from build123d import *

# Parameters (mm, degrees)
CUT_EXTRUDE1_DEPTH      = 64.162373268
CUT_EXTRUDE1_DEPTH_BACK = 64.162373268
SKETCH2_R               = 5
CUT_EXTRUDE2_DEPTH      = 63.964159794
CUT_EXTRUDE2_DEPTH_BACK = 63.964159794
SKETCH3_R               = 5


with BuildPart() as part:
    # Sketch1 → Revolve1 (revolve)
    with BuildSketch(Plane.XY, mode=Mode.PRIVATE) as revolve1_sk:
        Polygon((11.25, 0), (11.25, 12), (18, 12), (27.357798165, 42), (33.357798165, 42), (22.5, 0), align=None)
    revolve(revolve1_sk.sketch.rotate(Axis((0, 40.458715596, 0), (0, -1, 0)), 90), axis=Axis((0, 40.458715596, 0), (0, -1, 0)))

    # Sketch2 → Cut-Extrude1 (cut, two sides: drawn at the far end of the back side and taken through both)
    with BuildSketch(Plane.XY.offset(-CUT_EXTRUDE1_DEPTH_BACK)):
        with Locations((0, 42)):
            Circle(SKETCH2_R)
    extrude(amount=CUT_EXTRUDE1_DEPTH + CUT_EXTRUDE1_DEPTH_BACK, mode=Mode.SUBTRACT)

    # Sketch3 → Cut-Extrude2 (cut, two sides: drawn at the far end of the back side and taken through both)
    with BuildSketch(Plane(origin=(0, 0, 0), x_dir=(0, 0, -1), z_dir=(1, 0, 0)).offset(-CUT_EXTRUDE2_DEPTH_BACK)):
        with Locations((0, 42)):
            Circle(SKETCH3_R)
    extrude(amount=CUT_EXTRUDE2_DEPTH + CUT_EXTRUDE2_DEPTH_BACK, mode=Mode.SUBTRACT)


solid = part.part
Model file for the job. Use its own axes, mm. Give positions to 0.01 mm unless a question says otherwise; leave off trailing zeros. Order: outer loops, then holes, each group sorted by start corner. A loop starts at its lowest first (then second) coordinate and runs counter-clockwise, first axis right, second up. Notation, with made-up numbers: M -19,-33.5 L 30,-33.5 A32 ccw 30,2.5 Z; hole C -12.5,-29 d10. An arc over 180 degrees is marked long. Put each result on its own line as item: value. Start each with the question number.
(1) Band-saw the part on D-D on y = 32. Give the cut face in (x, z), then the cut area to 3 significant figures.
(2) Pin check, flat tips, straight feed: pin 1 Ø4 at (x, y) = (10, 22) entering from +Z; pin 2 Ø10 at (y, z) = (7, 1.5) entering from +X; pin 3 Ø3 at (y, z) = (12.5, -17) entering from -X. Stop position of each tip, or through.
(3) Pull direction Z, two halves, no side cores. Call faces 1 (the face through (-21, 42, -20)), 2 (the face through (12, 12, 0)), 3 (the face through (-8.004, 16.039, 25.416)), 4 (the face through (-29, 37, 0)): released by +Z, released by -Z, zero draft, split by the parting line, or undercut.
(4) Band-saw the part on C-C on y = 10.5. Give the cut face in (x, z).
(5) Drill centre lines: L1, parallel to Y at x = 12.5, z = 1.5; L2, parallel to Z at x = 4, y = 22.5; L3, parallel to Z at x = 3, y = 35.5. Where is each one in solid material? Low to high. Write a range as [from, to].
(6) Band-saw the part on A-A on z = 0. Give the cut face in (x, y).
(7) Band-saw the part on B-B on x = 0. Give the cut face in (y, z), then the cut area to 3 significant figures.
Results below:
1. outline: C 0,0 d61.55; hole C 0,0 d48.48
1. area: 1,130 mm2
2. pin 1: stops at z = 27.23
2. pin 2: stops at x = 25.58
2. pin 3: stops at x = -20.64
3. face 1: zero draft
3. face 2: undercut
3. face 3: split by the parting line
3. face 4: undercut
4. outline: C 0,0 d50.43; hole C 0,0 d22.5
5. L1: y = [0, 12]
5. L2: z = [-28.03, -20.9], [20.9, 28.03]
5. L3: z = [-31.54, -25.15], [25.15, 31.54]
6. outline: M -32.07,37 L -22.5,0 L -11.25,0 L -11.25,12 L -18,12 L -25.8,37 Z; M 11.25,0 L 22.5,0 L 32.07,37 L 25.8,37 L 18,12 L 11.25,12 Z
7. outline: M 0,-22.5 L 37,-32.07 L 37,-25.8 L 12,-18 L 12,-11.25 L 0,-11.25 Z; M 0,11.25 L 12,11.25 L 12,18 L 37,25.8 L 37,32.07 L 0,22.5 Z
7. area: 654 mm2
